CAD build for the part. Positions are in the model's coordinates, mm. A direction names the side the tool comes from. Coordinates: 2 decimals unless noted, no trailing zeros. Order: outer loops, then holes, each group sorted by start corner. A loop starts at its lowest first (then second) coordinate and runs counter-clockwise, first axis right, second up. Notation, with made-up numbers: M 77.5,50.5 L 98.5,50.5 A21 ccw 98.5,63.5 Z; hole C 14,-32.75 d5. An arc over 180 degrees is marked long. Write item = value, one per line.
from build123d import *

# Parameters (mm, degrees)
SKETCH1_W             = 12
SKETCH1_H             = 12
BOSS_EXTRUDE1_DEPTH   = 7
SKETCH2_W             = 0.5
SKETCH2_H             = 1.5
BOSS_EXTRUDE2_DEPTH   = 4
SKETCH2_W_2           = 2
SKETCH2_H_2           = 0.5
BOSS_EXTRUDE2_2_DEPTH = 4
BOSS_EXTRUDE2_3_DEPTH = 4
BOSS_EXTRUDE2_4_DEPTH = 4
BOSS_EXTRUDE2_5_DEPTH = 4
BOSS_EXTRUDE2_6_DEPTH = 4
BOSS_EXTRUDE2_7_DEPTH = 4
SKETCH3_W             = 13
SKETCH3_H             = 13
SKETCH3_W_2           = 12
SKETCH3_H_2           = 12
BOSS_EXTRUDE3_DEPTH   = 7
SKETCH4_R             = 3.25
BOSS_EXTRUDE4_DEPTH   = 7.5
SKETCH5_R             = 3
BOSS_EXTRUDE5_DEPTH   = 13
CUT_EXTRUDE1_START    = -10
CUT_EXTRUDE1_DEPTH    = 10


with BuildPart() as part:
    # Sketch1 → Boss-Extrude1 (new body)
    with BuildSketch(Plane(origin=(0, 0, 0), x_dir=(1, 0, 0), z_dir=(0, 1, 0))):
        with Locations((-6, -6)):
            Rectangle(SKETCH1_W, SKETCH1_H)
    extrude(amount=BOSS_EXTRUDE1_DEPTH)



with BuildPart() as body_2:
    # Sketch2 → Boss-Extrude2 (new body)
    with BuildSketch(Plane.XZ):
        with Locations((-12.25, 9.25)):
            Rectangle(SKETCH2_W, SKETCH2_H)
    extrude(amount=BOSS_EXTRUDE2_DEPTH)


with BuildPart() as body_3:
    # Sketch2 → Boss-Extrude2 2 (new body)
    with BuildSketch(Plane.XZ):
        with Locations((-6, -0.25)):
            Rectangle(SKETCH2_W_2, SKETCH2_H_2)
    extrude(amount=BOSS_EXTRUDE2_2_DEPTH)


with BuildPart() as body_4:
    # Sketch2 → Boss-Extrude2 3 (new body)
    with BuildSketch(Plane.XZ):
        with Locations((0.25, 2.75)):
            Rectangle(SKETCH2_W, SKETCH2_H)
    extrude(amount=BOSS_EXTRUDE2_3_DEPTH)


with BuildPart() as body_5:
    # Sketch2 → Boss-Extrude2 4 (new body)
    with BuildSketch(Plane.XZ):
        with Locations((-6, 12.25)):
            Rectangle(SKETCH2_W_2, SKETCH2_H_2)
    extrude(amount=BOSS_EXTRUDE2_4_DEPTH)


with BuildPart() as body_6:
    # Sketch2 → Boss-Extrude2 5 (new body)
    with BuildSketch(Plane.XZ):
        with Locations((-12.25, 6.043)):
            Rectangle(SKETCH2_W, SKETCH2_H)
    extrude(amount=BOSS_EXTRUDE2_5_DEPTH)


with BuildPart() as body_7:
    # Sketch2 → Boss-Extrude2 6 (new body)
    with BuildSketch(Plane.XZ):
        with Locations((-12.25, 2.75)):
            Rectangle(SKETCH2_W, SKETCH2_H)
    extrude(amount=BOSS_EXTRUDE2_6_DEPTH)


with BuildPart() as body_8:
    # Sketch2 → Boss-Extrude2 7 (new body)
    with BuildSketch(Plane.XZ):
        with Locations((0.25, 9.25)):
            Rectangle(SKETCH2_W, SKETCH2_H)
    extrude(amount=BOSS_EXTRUDE2_7_DEPTH)


with BuildPart() as part_1:
    add(part.part)

    add(body_2.part)  # Boss-Extrude3 merges body 2

    add(body_3.part)  # Boss-Extrude3 merges body 3

    add(body_4.part)  # Boss-Extrude3 merges body 4

    add(body_5.part)  # Boss-Extrude3 merges body 5

    add(body_6.part)  # Boss-Extrude3 merges body 6

    add(body_7.part)  # Boss-Extrude3 merges body 7

    add(body_8.part)  # Boss-Extrude3 merges body 8
    # Sketch3 → Boss-Extrude3 (add)
    with BuildSketch(Plane(origin=(0, 7, 0), x_dir=(1, 0, 0), z_dir=(0, 1, 0))):
        with Locations((-6, -6)):
            Rectangle(SKETCH3_W, SKETCH3_H)
        with Locations((-6, -6)):
            Rectangle(SKETCH3_W_2, SKETCH3_H_2, mode=Mode.SUBTRACT)
    extrude(amount=-BOSS_EXTRUDE3_DEPTH)

    # Sketch4 → Boss-Extrude4 (add)
    with BuildSketch(Plane(origin=(0, 7, 0), x_dir=(1, 0, 0), z_dir=(0, 1, 0))):
        with Locations(Location((-6, -6, 0), (0, 0, 270))):
            Circle(SKETCH4_R)
    extrude(amount=BOSS_EXTRUDE4_DEPTH)

    # Sketch5 → Boss-Extrude5 (add)
    with BuildSketch(Plane(origin=(0, 14.5, 0), x_dir=(1, 0, 0), z_dir=(0, 1, 0))):
        with Locations(Location((-6, -6, 0), (0, 0, 90))):
            Circle(SKETCH5_R)
    extrude(amount=BOSS_EXTRUDE5_DEPTH)

    # Sketch6 → Cut-Extrude1 (cut)
    with BuildSketch(Plane(origin=(0, 27.5, 0), x_dir=(1, 0, 0), z_dir=(0, 1, 0)).offset(CUT_EXTRUDE1_START)):
        with BuildLine():
            Line((-8.828427125, -7), (-3.171572875, -7))
            ThreePointArc((-3.171572875, -7), (-6, -9), (-8.828427125, -7))
        make_face()
    extrude(amount=CUT_EXTRUDE1_DEPTH, mode=Mode.SUBTRACT)


solid = part_1.part
(1) Slice it at D-D, the plane z = 10.5. Write the cut outline in (x, y).
Evaluation:
outline = M -12.5,0 L 0.5,0 L 0.5,7 L -12.5,7 Z
(2) Wall check: line 1 (X direction, y = -2, z = 2.5); line 2 (Y direction, x = -3.5, z = 11.75); line 3 (Y direction, x = -6.75, z = 3.5). Give the ranges that are in metal, low to high. Write a range as from..to.
Evaluation:
line_1 = -12.5..-12, 0..0.5
line_2 = 0..7
line_3 = 0..27.5
(3) Tool access for faces 4 (the face through (-5.02, 10.7, 9.1)), 5 (the face through (-6, -2, 0)), 6 (the face through (-6, 17.5, 8)), 7 (the face through (-12, -2, 6)): list every direction of +Z, -Z, +X, -X, +Y, -Y with a clear straight run to the whole face (end or side of a thin tool).
Evaluation:
face_4 = +Y
face_5 = +X, -X, -Y
face_6 = +Z, +X, -X, +Y
face_7 = +Z, -Z, +X, -Y
(4) Slice it at A-A, the plane y = -1. Write the cut outline in (x, z).
Evaluation:
outline = M -12.5,2 L -12,2 L -12,3.5 L -12.5,3.5 Z; M -12.5,5.29 L -12,5.29 L -12,6.79 L -12.5,6.79 Z; M -12.5,8.5 L -12,8.5 L -12,10 L -12.5,10 Z; M -7,-0.5 L -5,-0.5 L -5,0 L -7,0 Z; M -7,12 L -5,12 L -5,12.5 L -7,12.5 Z; M 0,2 L 0.5,2 L 0.5,3.5 L 0,3.5 Z; M 0,8.5 L 0.5,8.5 L 0.5,10 L 0,10 Z
(5) Slice it at C-C, the plane x = -6. Write the cut outline in (y, z).
Evaluation:
outline = M -4,-0.5 L 7,-0.5 L 7,2.75 L 14.5,2.75 L 14.5,3 L 27.5,3 L 27.5,7 L 17.5,7 L 17.5,9 L 14.5,9 L 14.5,9.25 L 7,9.25 L 7,12.5 L -4,12.5 L -4,12 L 0,12 L 0,0 L -4,0 Z
(6) Pin check, flat tips, straight feed: pin 1 Ø3 at (x, y) = (-7, 23) entering from +Z; pin 2 Ø0.6 at (x, z) = (-5, 8) entering from +Y; pin 3 Ø5 at (y, z) = (17.5, 2.5) entering from +X. Stop position of each tip, or through.
Evaluation:
pin_1 = 7
pin_2 = 17.5
pin_3 = -3.17
(7) Pull direction Z, two halves, no side cores. Call faces 1 (the face through (-4.85, 20.91, 3.23)), 2 (the face through (-12, -2, 9)), 3 (the face through (-6, -2, 12)): +Z half, -Z half, draft (parallel to the pull), parting line (faces both ways), or undercut.
Evaluation:
face_1 = parting line
face_2 = draft
face_3 = undercut
(8) Slice it at B-B, the plane z = 6. Write the cut outline in (x, y).
Evaluation:
outline = M -12.5,-4 L -12,-4 L -12,0 L 0.5,0 L 0.5,7 L -2.75,7 L -2.75,14.5 L -3,14.5 L -3,27.5 L -9,27.5 L -9,14.5 L -9.25,14.5 L -9.25,7 L -12.5,7 Z
